Here's how the part is built. I have some questions about the finished solid (model axes, mm). Face numbers are marked on the shaded views. A direction names the side the tool comes from. Coordinates: 2 decimals unless noted, no trailing zeros. Write each loop counter-clockwise with the first axis right and the second up, starting at its lowest first coordinate (ties: lowest second). Pieces come first, ordered by that corner, then holes.
```python
from build123d import *

# Parameters (mm, degrees)
COIL_START = -0.7
SKETCH1_W  = 2.6
SKETCH1_H  = 10
COIL_DEPTH = 8.5
FILLET1_R  = 0.1


with BuildPart() as part:
    # Sketch1 → Coil (new body)
    with BuildSketch(Plane(origin=(0, 97.279475289, 0), x_dir=(1, 0, 0), z_dir=(0, 1, 0)).offset(COIL_START)):
        with BuildLine():
            Line((87.072792821, 67.609367759), (91.072792821, 67.609367759))
            ThreePointArc((91.072792821, 67.609367759), (92.487006384, 68.195154196), (93.072792821, 69.609367759))
            Line((93.072792821, 69.609367759), (93.072792821, 78.609367759))
            ThreePointArc((93.072792821, 78.609367759), (92.487006384, 80.023581321), (91.072792821, 80.609367759))
            Line((91.072792821, 80.609367759), (87.072792821, 80.609367759))
            ThreePointArc((87.072792821, 80.609367759), (85.658579259, 80.023581321), (85.072792821, 78.609367759))
            Line((85.072792821, 78.609367759), (85.072792821, 69.609367759))
            ThreePointArc((85.072792821, 69.609367759), (85.658579259, 68.195154196), (87.072792821, 67.609367759))
        make_face()
        with Locations((89.072792821, 74.109367759)):
            Rectangle(SKETCH1_W, SKETCH1_H, mode=Mode.SUBTRACT)
    extrude(amount=-COIL_DEPTH)

    # Fillet1
    fillet1_edges = [part.edges().sort_by_distance(p)[0] for p in [
        (90.372792821, 92.329475289, -79.109367759),
        (90.372792821, 92.329475289, -69.109367759),
        (87.772792821, 92.329475289, -69.109367759),
        (87.772792821, 92.329475289, -79.109367759),
    ]]
    fillet(fillet1_edges, radius=FILLET1_R)


solid = part.part
```
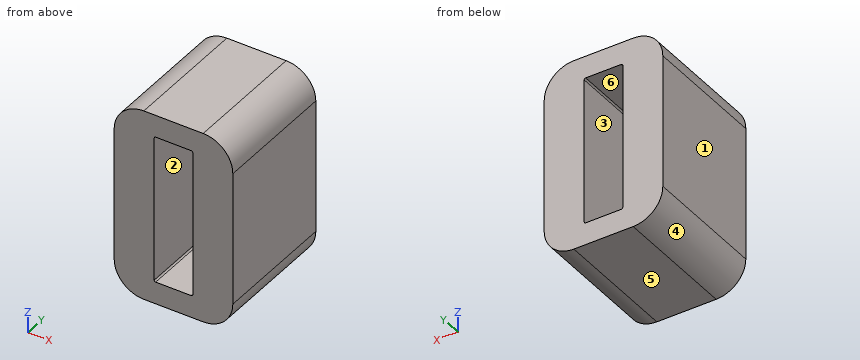
1) We'd pull the mould along X, two halves only. Please class the marked faces 3, 4, 5 and 6: pulls with the +X half, pulls with the -X half, needs draft (parallel to the pull), parting line crosses it, or undercut.
Values follow:
face 3: undercut
face 4: pulls with the -X half
face 5: needs draft
face 6: undercut
2) On a 3-axis mill with a long thin cutter (end or side, diameter ignored), from which of +Z, -Z, +X, -X, +Y, -Y can I reach the whole of each face in a straight line? I mean the marked faces 1 and 2. Say none if no direction works.
Values follow:
face 1: +Z, -Z, -X, +Y, -Y
face 2: +Y, -Y
3) Imagine slicing it at D-D on x = 92.5. Please give me the cut outline in (y, z), then the cut area to 3 significant figures.
Values follow:
outline: (88.08, -80.01) - (96.58, -80.01) - (96.58, -68.21) - (88.08, -68.21) - close
area: 100 mm2
4) Imagine slicing it at C-C on x = 89.5. Please give me the cut outline in (y, z), then the cut area to 3 significant figures.
Values follow:
outline: (88.08, -80.61) - (96.58, -80.61) - (96.58, -79.11) - (88.08, -79.11) - close; (88.08, -69.11) - (96.58, -69.11) - (96.58, -67.61) - (88.08, -67.61) - close
area: 25.5 mm2
5) Imagine slicing it at B-B on z = -70.75. Please give me the cut outline in (x, y).
Values follow:
outline: (85.07, 88.08) - (87.77, 88.08) - (87.77, 96.58) - (85.07, 96.58) - close; (90.37, 88.08) - (93.07, 88.08) - (93.07, 96.58) - (90.37, 96.58) - close
6) I need wall thicknesses on probe 1 along X at (y, z) = (92.25, -78.25); probe 2 along Z at (x, y) = (90, 92.75); probe 3 along Z at (x, y) = (91.5, 94.75). Which ranges of each line are inside material? Lowest first, please.
Values follow:
probe 1: x = 85.07 to 87.77, 90.37 to 93.07
probe 2: z = -80.61 to -79.11, -69.11 to -67.61
probe 3: z = -80.56 to -67.66
7) Imagine slicing it at A-A on y = 95.5. Please give me the cut outline in (x, z).
Values follow:
outline: (85.07, -78.61) arc R2 ccw to (87.07, -80.61) - (91.07, -80.61) arc R2 ccw to (93.07, -78.61) - (93.07, -69.61) arc R2 ccw to (91.07, -67.61) - (87.07, -67.61) arc R2 ccw to (85.07, -69.61) - close; hole (87.77, -79.01) arc R0.1 ccw to (87.87, -79.11) - (90.27, -79.11) arc R0.1 ccw to (90.37, -79.01) - (90.37, -69.21) arc R0.1 ccw to (90.27, -69.11) - (87.87, -69.11) arc R0.1 ccw to (87.77, -69.21) - close
